The model under review builds one solid part; all positions refer to its coordinate system, in mm. Round coordinates to 2 decimals unless told otherwise and drop trailing zeros. Loops run counter-clockwise (first coordinate to the right, second up) from the corner with the lowest first, then second, coordinate; pieces in that order, holes last. Notation, with made-up numbers: (46.25, -39.5) -> (54.25, -39.5) arc R17 ccw to (54.25, -11.5) -> close; hole circle Ø8 at (1, -3). An arc over 180 degrees is marked (long way). Use a Markdown table: item, result. Add a question column.
1) Consider section B-B on x = 57.25. Give the boundary of the cut face in (y, z).
2) Consider section D-D on y = 21.5. Give the boundary of the cut face in (x, z), plus the area to 3 significant figures.
3) Consider section C-C on z = -51. Give the boundary of the cut face in (x, y).
4) Consider section A-A on y = 13. Give the boundary of the cut face in (x, z), plus the area to 3 significant figures.
5) Insertion check: pin 1 (4 mm diameter, centred on x = 50.5, z = -46, fed in from -Y); pin 2 (1 mm diameter, centred on x = 52.5, z = -13.5, fed in from +Y); pin 3 (12 mm diameter, centred on y = 19, z = -87, fed in from +X). Each pin has a flat end and moves straight along its axis. Give the tip position at first contact, or say it passes through.
6) Wall thickness on probe 1 along Z at (x, y) = (54.25, 12.25); probe 2 along X at (y, z) = (18.25, -79.5); probe 3 along X at (y, z) = (16.75, -20): over which ranges is each line inside the solid? List them lowest first.
Autodesk Inventor part; units mm, degrees
ref_plane "Work Plane1" through (0, 0, -97.5) normal (0, 0, -1) x (0, 1, 0)
ref_plane "YZ Plane" through (0, 0, 0) normal (1, 0, 0) x (0, 1, 0)
ref_plane "XZ Plane" through (0, 0, 0) normal (0, 1, 0) x (-1, 0, 0)
sketch "Sketch1" plane through (0, 0, 0) normal (0, 0, 1) x (1, 0, 0)
  line L0 (44.9961, 27) -> (47.3055, 27)
  line L1 (47.3055, 27) -> (61.6238, 2.2)
  line L2 (61.6238, 2.2) -> (59.3144, 2.2)
  line L3 (59.3144, 2.2) -> (44.9961, 27) construction
  line L4 (44.9961, 27) -> (59.3144, 2.2)
  line L5 (16.5, 27) -> (44.9961, 27) construction
  point P0 (0, 0)
  dimension "d10" = 2
ref_plane "Work Plane1" through (0, 0, -97.5) normal (0, 0, -1) x (0, 1, 0)
extrude "Extrusion1" add sketch "Sketch1" against normal up to surface (97.5 mm away)
sketch "Sketch2" plane through (47.3055, 27, 0) normal (0.8660254, 0.5, 0) x (0, 0, -1)
  line L0 (15.75, -28.6366) -> (37.75, -28.6366)
  line L1 (37.75, -28.6366) -> (37.75, -11.6366)
  line L2 (37.75, -11.6366) -> (15.75, -11.6366)
  line L3 (15.75, -11.6366) -> (15.75, -28.6366)
  line L4 (0, 0) -> (97.5, 0) construction
  line L5 (48.75, 0) -> (48.75, -28.6366) construction
  line L6 (0, -28.6366) -> (97.5, -28.6366) construction
  line L7 (81.75, -28.6366) -> (59.75, -28.6366)
  line L8 (59.75, -28.6366) -> (59.75, -11.6366)
  line L9 (59.75, -11.6366) -> (81.75, -11.6366)
  line L10 (81.75, -11.6366) -> (81.75, -28.6366)
  point P0 (0, 0.2701)
  dimension "d4" = 22
  dimension "d5" = 22
  dimension "d6" = 17
extrude "Extrusion2" cut sketch "Sketch2" against normal through all
fillet "Fillet1" radius 2 4 edges at (52.2577, 16.4224, -37.75) (52.2577, 16.4224, -15.75) (52.2577, 16.4224, -59.75) (52.2577, 16.4224, -81.75)
properties part number "Przod" material "Aluminum 6061"
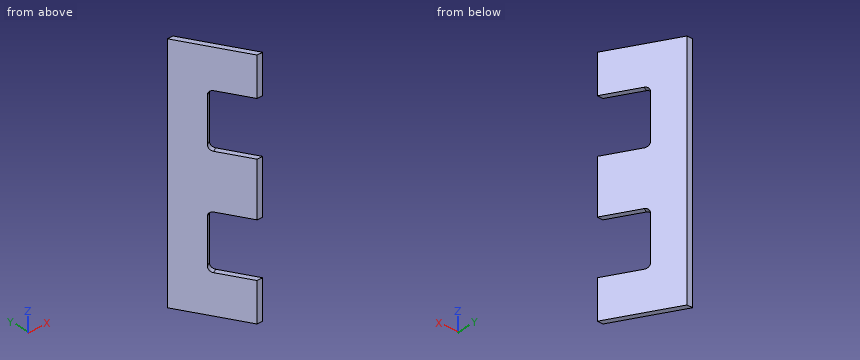
Result set:
| question | item | result |
|---|---|---|
| 1 | outline | (5.78, -97.5) -> (9.78, -97.5) -> (9.78, -81.75) -> (5.78, -81.75) -> close; (5.78, -59.75) -> (9.78, -59.75) -> (9.78, -37.75) -> (5.78, -37.75) -> close; (5.78, -15.75) -> (9.78, -15.75) -> (9.78, 0) -> (5.78, 0) -> close |
| 2 | outline | (48.17, -97.5) -> (50.48, -97.5) -> (50.48, 0) -> (48.17, 0) -> close |
| 2 | area | 225 mm2 |
| 3 | outline | (45, 27) -> (59.31, 2.2) -> (61.62, 2.2) -> (47.31, 27) -> close |
| 4 | outline | (53.08, -97.5) -> (55.39, -97.5) -> (55.39, -81.75) -> (53.08, -81.75) -> close; (53.08, -59.75) -> (55.39, -59.75) -> (55.39, -37.75) -> (53.08, -37.75) -> close; (53.08, -15.75) -> (55.39, -15.75) -> (55.39, 0) -> (53.08, 0) -> close |
| 4 | area | 124 mm2 |
| 5 | pin 1 | y = 14 |
| 5 | pin 2 | y = 18.87 |
| 5 | pin 3 | x = 55.39 |
| 6 | probe 1 | -97.5 to -81.75, -59.75 to -37.75, -15.75 to 0 |
| 6 | probe 2 | 50.05 to 52.36 |
| 6 | probe 3 | 50.91 to 52.83 |
